Can you work these out from the drawing? Everything is in mm from the part's minimum corner. Round coordinates to 2 decimals unless told otherwise and drop trailing zeros. Loops run counter-clockwise (first coordinate to the right, second up) from the corner with the lowest first, then second, coordinate; pieces in that order, holes last. Notation, with made-up numbers: (-3, 34.5) - (34, 34.5) arc R24 cw to (34, 62.5) - close; hole circle Ø10 at (63.5, -36.75). An arc over 180 degrees is marked (long way). Answer as a JSON object with one key per item and string values. Group by question number.
1) If we mould it in two halves opening along Z, with no side actions, what happens to the marked faces 1, 2 and 3? For each: pulls with the +Z half, pulls with the -Z half, needs draft (parallel to the pull), parting line crosses it, or undercut.
2) I want a section at A-A, the plane x = 31.75. Please give me the cut outline in (y, z).
3) I want a section at D-D, the plane x = 19.5. Please give me the cut outline in (y, z), then the cut area to 3 significant figures.
4) Will these pins go through, and if not, where does the flat tip stop? P1, Ø3.5, axis at x = 31.75, y = 31.75, coming from the +Z side; P2, Ø5, axis at x = 38, z = 14, coming from the -Y side; P3, Ø2.5, axis at x = 32.5, z = 15, coming from the -Y side; P4, Ø5, axis at x = 16.5, z = 15, coming from the -Y side.
5) I want a section at B-B, the plane y = 31.75. Please give me the cut outline in (x, z), then the cut area to 3 significant figures.
6) If I drill on line 1 along X through (y, z) = (31.75, 4.5); line 2 along X through (y, z) = (31.75, 11.5); line 3 along Y through (x, z) = (31.75, 15.75), over which ranges is the centre line in solid material (lowest first)? Write a range as [from, to].
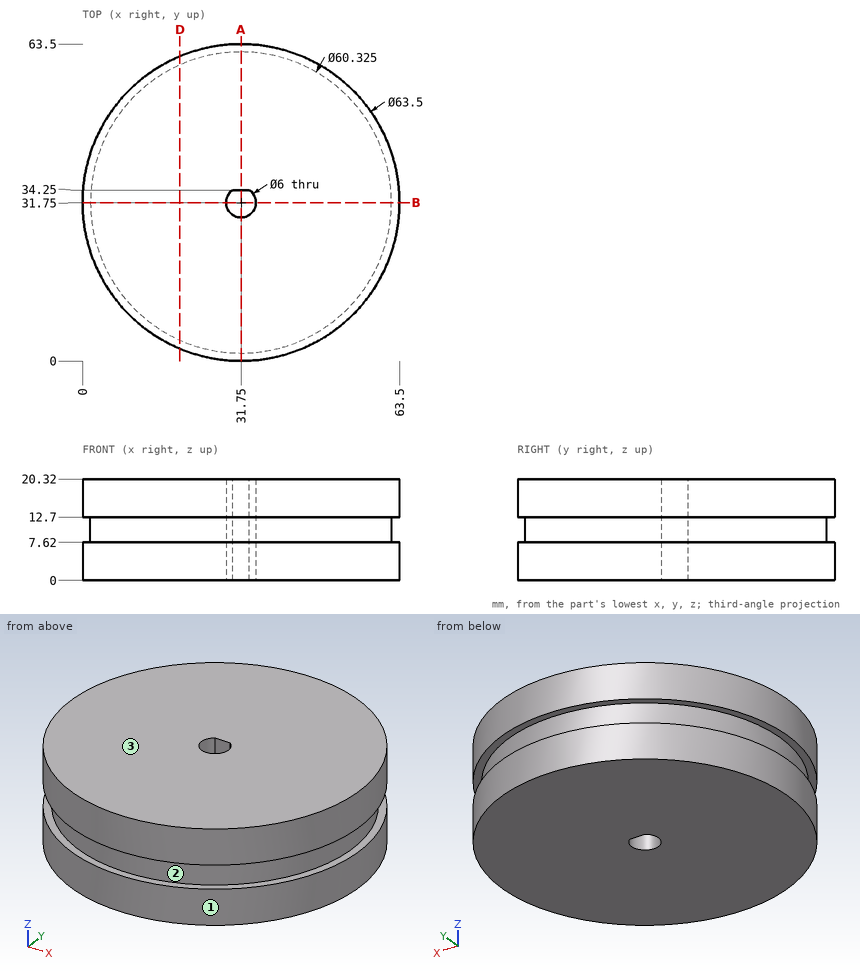
Outcome:
{
 "1": {"face 1": "needs draft", "face 2": "undercut", "face 3": "pulls with the +Z half"},
 "2": {"outline": "(0, 0) - (28.75, 0) - (28.75, 20.32) - (0, 20.32) - (0, 12.7) - (1.59, 12.7) - (1.59, 7.62) - (0, 7.62) - close; (34.25, 0) - (63.5, 0) - (63.5, 7.62) - (61.91, 7.62) - (61.91, 12.7) - (63.5, 12.7) - (63.5, 20.32) - (34.25, 20.32) - close"},
 "3": {"outline": "(2.46, 0) - (61.04, 0) - (61.04, 7.62) - (59.31, 7.62) - (59.31, 12.7) - (61.04, 12.7) - (61.04, 20.32) - (2.46, 20.32) - (2.46, 12.7) - (4.19, 12.7) - (4.19, 7.62) - (2.46, 7.62) - close", "area": "1,170 mm^2"},
 "4": {"P1": "through", "P2": "y = 0.22", "P3": "y = 0", "P4": "y = 2.67"},
 "5": {"outline": "(0, 0) - (28.75, 0) - (28.75, 20.32) - (0, 20.32) - (0, 12.7) - (1.59, 12.7) - (1.59, 7.62) - (0, 7.62) - close; (34.75, 0) - (63.5, 0) - (63.5, 7.62) - (61.91, 7.62) - (61.91, 12.7) - (63.5, 12.7) - (63.5, 20.32) - (34.75, 20.32) - close", "area": "1,150 mm^2"},
 "6": {"line 1": "[0, 28.75], [34.75, 63.5]", "line 2": "[1.59, 28.75], [34.75, 61.91]", "line 3": "[0, 28.75], [34.25, 63.5]"}
}
